Build history of the part. All positions in model axes, mm. A direction names the side the tool comes from. Round coordinates to 2 decimals unless told otherwise and drop trailing zeros. Write each loop counter-clockwise with the first axis right and the second up, starting at its lowest first coordinate (ties: lowest second). Pieces come first, ordered by that corner, then holes. Notation, with made-up numbers: (-7.75, -15.5) -> (9.25, -15.5) arc R28 ccw to (9.25, 21.5) -> close; hole circle Ø1 at (63.5, 52.25). An arc over 180 degrees is marked (long way). Return JSON: item names as keys, results as strings.
from build123d import *

# Parameters (mm, degrees)
SKETCH1_R                = 3
BOSS_EXTRUDE1_DEPTH      = 20
SKETCH2_R                = 3.770107986
SKETCH2_R_2              = 2.770107986
EXTRUDE_THIN1_DEPTH      = 1
EXTRUDE_THIN1_DEPTH_BACK = 2


with BuildPart() as part:
    # Sketch1 → Boss-Extrude1 (new body)
    with BuildSketch(Plane.XY):
        Circle(SKETCH1_R)
    extrude(amount=BOSS_EXTRUDE1_DEPTH)

    # Sketch2 → Extrude-Thin1 (add, two sides)
    with BuildSketch(Plane(origin=(0, 0, 0), x_dir=(-1, 0, 0), z_dir=(0, 0, -1))) as extrude_thin1_sk:
        Circle(SKETCH2_R)
        Circle(SKETCH2_R_2, mode=Mode.SUBTRACT)
    extrude(amount=EXTRUDE_THIN1_DEPTH)
    extrude(extrude_thin1_sk.sketch, amount=-EXTRUDE_THIN1_DEPTH_BACK)


solid = part.part
Q1. Saw through at D-D on x = 3.25. List the corners of the cut face in (y, z), then the cut area to 3 significant figures.
Verdict:
{"outline": "(-1.91, -1) -> (1.91, -1) -> (1.91, 2) -> (-1.91, 2) -> close", "area": "11.5 mm²"}
Q2. Two-plate mould, pull along Y, no slides. Class faces 1 (the flat face through (0, 0, 20)), 2 (the cylindrical face through (3.766, 0.166, 0.479)), 3 (the cylindrical face through (-2.642, 0.832, -0.493)): +Y half, -Y half, draft (parallel to the pull), parting line (faces both ways), or undercut.
Verdict:
{"face 1": "draft", "face 2": "parting line", "face 3": "undercut"}
Q3. 3-axis set-ups, long thin cutter, end or side, ignore diameter. For faces 4 (the flat face through (0, 3, -1)), 5 (the flat face through (3, -2, 2)), 6 (the flat face through (0, 0, 0)): which of +Z, -Z, +X, -X, +Y, -Y reach the whole face in a straight line?
Verdict:
{"face 4": "-Z, +X, -X, +Y, -Y", "face 5": "+Z", "face 6": "-Z"}
Q4. Wall check: L1, parallel to Y at x = 0, z = -0.8; L2, parallel to Z at x = 1.5, y = 2; L3, parallel to Z at x = 3.5, y = -0.75. Give the ranges that are in metal, low to high.
Verdict:
{"L1": "y = -3.77 to -2.77, 2.77 to 3.77", "L2": "z = 0 to 20", "L3": "z = -1 to 2"}
Q5. Saw through at C-C on z = 12.75. List the corners of the cut face in (x, y), then the cut area to 3 significant figures.
Verdict:
{"outline": "circle Ø6 at (0, 0)", "area": "28.3 mm²"}
Q6. Saw through at A-A on x = 0. List the corners of the cut face in (y, z), then the cut area to 3 significant figures.
Verdict:
{"outline": "(-3.77, -1) -> (-2.77, -1) -> (-2.77, 0) -> (2.77, 0) -> (2.77, -1) -> (3.77, -1) -> (3.77, 2) -> (3, 2) -> (3, 20) -> (-3, 20) -> (-3, 2) -> (-3.77, 2) -> close", "area": "125 mm²"}
Q7. Pin check, flat tips, straight feed: pin 1 Ø1.7 at (x, y) = (-0.5, 0) entering from -Z; pin 2 Ø2 at (y, z) = (2, 4) entering from +X; pin 3 Ø3 at (x, z) = (-2.5, 14.5) entering from +Y. Stop position of each tip, or through.
Verdict:
{"pin 1": "stops at z = 0", "pin 2": "stops at x = 2.83", "pin 3": "stops at y = 2.83"}
